The listing builds one solid part. Answer for the finished solid, in the listing's coordinates (mm). A direction names the side the tool comes from. Round coordinates to 2 decimals unless told otherwise and drop trailing zeros. Write each loop counter-clockwise with the first axis right and the second up, starting at its lowest first coordinate (ties: lowest second). Pieces come first, ordered by that corner, then holes. Notation, with made-up numbers: (9, 26.5) - (65, 26.5) arc R31 cw to (65, 51.5) - close; hole circle Ø4 at (-15.75, -33). An arc over 180 degrees is marked (long way). Return JSON: item names as keys, results as strings. Group by question number.
from build123d import *

# Parameters (mm, degrees)
SKETCH1_W                      = 80
SKETCH1_H                      = 90
BOSS_EXTRUDE1_BASE_DEPTH       = 3
BOSS_EXTRUDE4_SIDE_WALLS_DEPTH = 90
CUT_EXTRUDE2_GUIDE_HOLES_DEPTH = 130.495173655
SKETCH15_W                     = 80
SKETCH15_H                     = 20
BOSS_EXTRUDE9_REAR_WALL_DEPTH  = 3
BOSS_EXTRUDE1_START            = 3
SKETCH17_W                     = 80
SKETCH17_H                     = 3
BOSS_EXTRUDE1_DEPTH            = 12
BOSS_EXTRUDE2_START            = 23
SKETCH20_W                     = 3
SKETCH20_H                     = 87
BOSS_EXTRUDE2_DEPTH            = 12
CHAMFER1_SIZE                  = 3
BOSS_EXTRUDE5_DEPTH            = 30
CHAMFER2_SIZE                  = 170.138454589
CHAMFER2_SIZE_2                = 30
SKETCH27_W                     = 80
SKETCH27_H                     = 91.38839507
BOSS_EXTRUDE6_DEPTH            = 3


# Some blends are built 0.0001 mm under size
with BuildPart() as part:
    # Sketch1 → Boss-Extrude1 _Base (new body)
    with BuildSketch(Plane(origin=(0, 0, 0), x_dir=(1, 0, 0), z_dir=(0, 1, 0))):
        with Locations((40, 45)):
            Rectangle(SKETCH1_W, SKETCH1_H)
    extrude(amount=BOSS_EXTRUDE1_BASE_DEPTH)

    # Sketch5 → Boss-Extrude4 _Side Walls (add, through all)
    with BuildSketch(Plane.XY):
        Polygon((-5, 28.390936655), (0, 38), (0, 0), (-5, 9.609063345), align=None)
        Polygon((85, 9.609063345), (85, 28.390936655), (80, 38), (80, 0), align=None)
    extrude(amount=-BOSS_EXTRUDE4_SIDE_WALLS_DEPTH)

    # Sketch4 → Cut-Extrude2 _Guide Holes (cut, through all)
    with BuildSketch(Plane.XY):
        Polygon((-3, 23), (0, 26), (0, 23), align=None)
        Polygon((80, 23), (83, 23), (80, 26), align=None)
    extrude(amount=-CUT_EXTRUDE2_GUIDE_HOLES_DEPTH, mode=Mode.SUBTRACT)

    # Sketch15 → Boss-Extrude9 _Rear Wall (add)
    with BuildSketch(Plane.XY):
        with Locations((40, 13)):
            Rectangle(SKETCH15_W, SKETCH15_H)
    extrude(amount=-BOSS_EXTRUDE9_REAR_WALL_DEPTH)

    # Sketch17 → Boss-Extrude1 (add)
    with BuildSketch(Plane(origin=(0, 23, 0), x_dir=(1, 0, 0), z_dir=(0, 1, 0)).offset(BOSS_EXTRUDE1_START)):
        with Locations((40, 1.5)):
            Rectangle(SKETCH17_W, SKETCH17_H)
    extrude(amount=BOSS_EXTRUDE1_DEPTH)

    # Sketch20 → Boss-Extrude2 (add)
    with BuildSketch(Plane(origin=(0, 3, 0), x_dir=(1, 0, 0), z_dir=(0, 1, 0)).offset(BOSS_EXTRUDE2_START)):
        with Locations((1.5, 46.5)):
            Rectangle(SKETCH20_W, SKETCH20_H)
        with Locations((78.5, 46.5)):
            Rectangle(SKETCH20_W, SKETCH20_H)
    extrude(amount=BOSS_EXTRUDE2_DEPTH)

    # Chamfer1
    chamfer1_edges = [part.edges().sort_by_distance(p)[0] for p in [
        (77, 26, -46.5),
        (3, 26, -46.5),
    ]]
    chamfer(chamfer1_edges, length=CHAMFER1_SIZE - 0.0001)  # a hair under: the kernel refuses the full size

    # Sketch26 → Boss-Extrude5 (add)
    with BuildSketch(Plane(origin=(0, 38, 0), x_dir=(1, 0, 0), z_dir=(0, 1, 0))):
        Polygon((77, 90), (80, 90), (80, 0), (0, 0), (0, 90), (3, 90), (3, 3), (77, 3), align=None)
    extrude(amount=BOSS_EXTRUDE5_DEPTH)

    # Chamfer2
    # the kernel refuses this chamfer: 170.138454589, 30 mm, written as the material it takes off along each edge
    with BuildSketch(Plane(origin=(522.111375011, 68, 0), x_dir=(0, 0.0066825316561015475, -0.9999776716360548), z_dir=(-1, 0, 0))) as chamfer2_piece_1:
        Polygon((CHAMFER2_SIZE * 0.999977671633, CHAMFER2_SIZE * 0.00668253165608), (-CHAMFER2_SIZE_2 * 0.0066825316561, CHAMFER2_SIZE_2 * 0.999977671636), (0, 0), align=None)
    extrude(amount=964.222750023, mode=Mode.SUBTRACT)

    # Sketch27 → Boss-Extrude6 (add)
    with BuildSketch(Plane(origin=(0, 36.854159795, 6.498382723), x_dir=(1, 0, 0), z_dir=(0, 0.9848077530122086, 0.17364817766692742))):
        with Locations((40, 52.292828286)):
            Rectangle(SKETCH27_W, SKETCH27_H)
    extrude(amount=-BOSS_EXTRUDE6_DEPTH)


solid = part.part
(1) Flat-ended cylindrical pins translate along their axes: pin 1 (5 mm diameter, centred on y = 48, z = -64, fed in from -X); pin 2 (3 mm diameter, centred on x = 32.5, y = 32.5, fed in from -Z); pin 3 (10 mm diameter, centred on x = 74.5, z = -10.5, fed in from +Y). Find the tip coordinate at first contact, or state that the pin passes through.
(2) Consider line 1 (X direction, y = 17, z = -69.5); line 2 (Z direction, x = 61.5, y = 22.5); line 3 (Y direction, x = 0.5, z = -63). Determine where each line is inside the solid, lowest interval first.
(3) Find section A-A (x = 56.5). Write down the section's boundary in (y, z) (3 decimals), plus the area to 3 significant figures.
(4) Find section C-C (y = 20). Write down the section's boundary in (x, z).
(5) Determine the mould class of faces 4 (the flat face through (1, 27, -46)), 5 (the flat face through (40.56, 46.046, -45.63)), 6 (the flat face through (0, 44, -55)), 7 (the flat face through (82.465, 4.737, -44.37)) for opening direction Y: +Y half, -Y half, draft (parallel to the pull), parting line (faces both ways), or undercut.
(6) For faces 1 (the flat face through (39, 13, -3)), 2 (the flat face through (39.8, 2.7, -90)), 3 (the flat face through (80, 44, -56)), determine the directions among +Z, -Z, +X, -X, +Y, -Y from which every point of the face is accessible in a straight line to the end or side of a thin tool.
Check sheet entries:
{
 "1": {"pin 1": "stops at x = 0", "pin 2": "stops at z = -3", "pin 3": "stops at y = 40.73"},
 "2": {"line 1": "x = -5 to 0, 80 to 85", "line 2": "z = -3 to 0", "line 3": "y = 0 to 3, 26.5 to 49.11"},
 "3": {"outline": "(0, -90) - (3, -90) - (3, -3) - (23, -3) - (23, 0) - (0, 0) - close; (26, -3) - (35.483, -3) - (50.915, -90.521) - (53.869, -90) - (38, 0) - (26, 0) - close", "area": "633 mm^2"},
 "4": {"outline": "(-5, -90) - (0, -90) - (0, -3) - (80, -3) - (80, -90) - (85, -90) - (85, 0) - (-5, 0) - close"},
 "5": {"face 4": "undercut", "face 5": "+Y half", "face 6": "draft", "face 7": "-Y half"},
 "6": {"face 1": "-Z", "face 2": "-Z, +X, -X, -Y", "face 3": "+Z, -Z, +X, +Y"}
}
